Job drawing, mm, ordinate dimensions from the low corner. One solid piece. Give positions to 0.01 mm unless a question says otherwise; leave off trailing zeros. Order: outer loops, then holes, each group sorted by start corner. A loop starts at its lowest first (then second) coordinate and runs counter-clockwise, first axis right, second up. Notation, with made-up numbers: (55, -3) - (86, -3) arc R12 ccw to (86, 9) - close; hole circle Ø4 at (61, 50). An arc over 180 degrees is marked (long way). Use one line per item in the form item = value. Start each with the question number.
1. Band-saw the part on A-A, the plane z = 0.4. List the corners of the cut face in (x, y).
2. Band-saw the part on C-C, the plane x = 7.5. List the corners of the cut face in (y, z).
3. Drill centre lines: line 1 (X direction, y = 0.5, z = 0.65); line 2 (Y direction, x = 4.25, z = 0.1); line 3 (Y direction, x = 8.75, z = 0.55). Where is each one in solid material? Low to high.
4. Pin check, flat tip, straight feed: P1, Ø1.5, axis at x = 6.5, y = 4, coming from the +Z side. Stop position of the tip, or through.
5. Band-saw the part on B-B, the plane y = 0.5. List the corners of the cut face in (x, z).
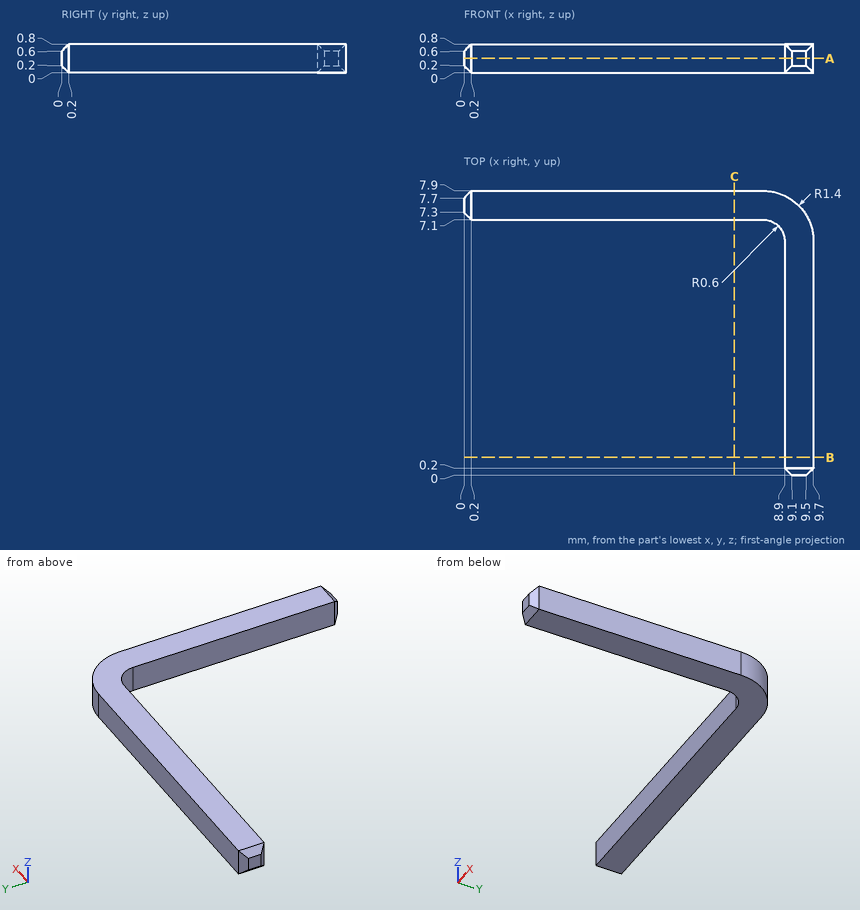
From the geometry:
q1.outline = (0, 7.3) - (0.2, 7.1) - (8.3, 7.1) arc R0.6 cw to (8.9, 6.5) - (8.9, 0.2) - (9.1, 0) - (9.5, 0) - (9.7, 0.2) - (9.7, 6.5) arc R1.4 ccw to (8.3, 7.9) - (0.2, 7.9) - (0, 7.7) - close
q2.outline = (7.1, 0) - (7.9, 0) - (7.9, 0.8) - (7.1, 0.8) - close
q3.line_1 = 8.9 to 9.7
q3.line_2 = 7.1 to 7.9
q3.line_3 = 6.9 to 7.83
q4.P1 = through
q5.outline = (8.9, 0) - (9.7, 0) - (9.7, 0.8) - (8.9, 0.8) - close
